Print and shaded views of the part. All mm, measured from the part's lowest x, y and z. Round coordinates to 2 decimals unless told otherwise and drop trailing zeros. Write each loop counter-clockwise with the first axis right and the second up, starting at its lowest first coordinate (ties: lowest second). Pieces come first, ordered by that corner, then holes.
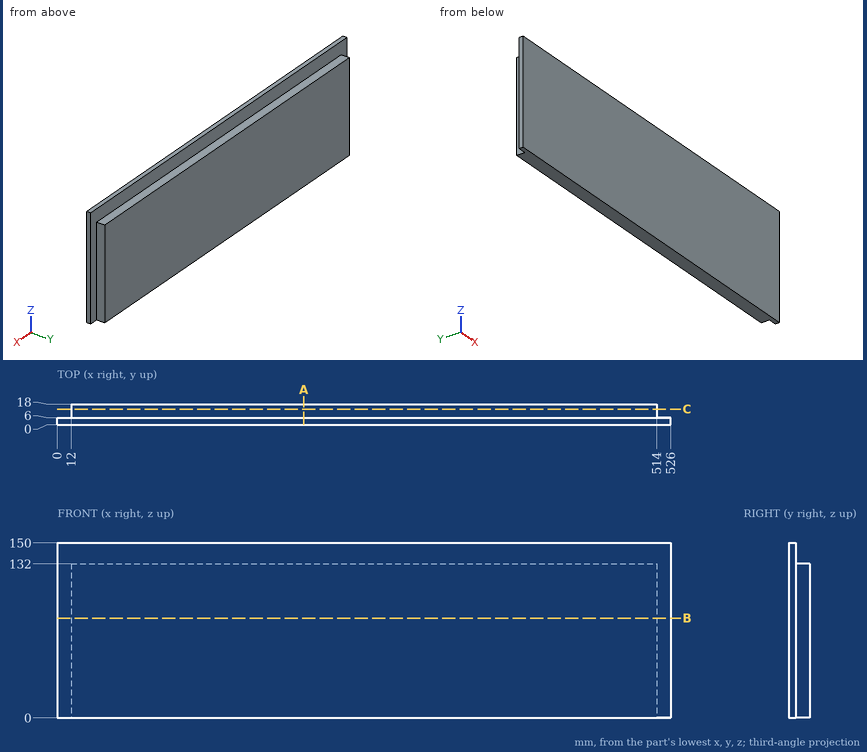
1) Slice it at C-C (y = 13.5). Write the cut outline in (x, z).
Results:
outline: (12, 0) - (514, 0) - (514, 132) - (12, 132) - close
2) Pin check, flat tips, straight feed: pin 1 Ø3.5 at (y, z) = (13, 87.5) entering from -X; pin 2 Ø5 at (y, z) = (9, 73) entering from +X; pin 3 Ø3.5 at (x, y) = (173.5, 13.5) entering from +Z. Stop position of each tip, or through.
Results:
pin 1: stops at x = 12
pin 2: stops at x = 514
pin 3: stops at z = 132
3) Slice it at B-B (z = 85.5). Write the cut outline in (x, y), plus the area to 3 significant figures.
Results:
outline: (0, 0) - (526, 0) - (526, 6) - (514, 6) - (514, 18) - (12, 18) - (12, 6) - (0, 6) - close
area: 9,180 mm2
4) Wall check: L1, parallel to Z at x = 84.5, y = 7.25; L2, parallel to X at y = 6.25, z = 22.5. Give the ranges that are in metal, low to high.
Results:
L1: z = 0 to 132
L2: x = 12 to 514
5) Slice it at A-A (x = 211.5). Write the cut outline in (y, z), plus the area to 3 significant figures.
Results:
outline: (0, 0) - (18, 0) - (18, 132) - (6, 132) - (6, 150) - (0, 150) - close
area: 2,480 mm2
